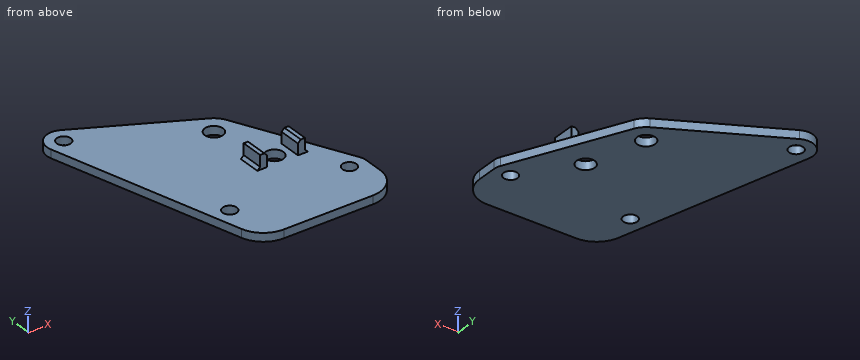
from build123d import *

# Parameters (mm, degrees)
SKETCH1_R           = 2.5
SKETCH1_R_2         = 3.25
BOSS_EXTRUDE1_DEPTH = 3
SKETCH2_W           = 2.5
SKETCH2_H           = 8
BOSS_EXTRUDE2_DEPTH = 5
CHAMFER1_SIZE       = 1
FILLET1_R           = 10


with BuildPart() as part:
    # Sketch1 → Boss-Extrude1 (new body)
    with BuildSketch(Plane.XY):
        with BuildLine():
            Line((-63.791318359, 58.43135993), (-43.395591792, -16.868352188))
            Line((-43.395591792, -16.868352188), (6, -16.868352188))
            Line((6, -16.868352188), (6, 0))
            ThreePointArc((6, 0), (5.850545761, 1.330832182), (5.409628568, 2.595364861))
            Line((5.409628568, 2.595364861), (-13.395576429, 41.791847675))
            ThreePointArc((-13.395576429, 41.791847675), (-14.765199318, 43.760307326), (-16.686113759, 45.195851809))
            Line((-16.686113759, 45.195851809), (-55.222801296, 65.318568168))
            ThreePointArc((-55.222801296, 65.318568168), (-61.758941161, 64.676575814), (-63.791318359, 58.43135993))
        make_face()
        Circle(SKETCH1_R, mode=Mode.SUBTRACT)
        with Locations((-58, 60)):
            Circle(SKETCH1_R, mode=Mode.SUBTRACT)
        with Locations((-42, 0.929027955)):
            Circle(SKETCH1_R, mode=Mode.SUBTRACT)
        with Locations((-20.157612139, 38.547641599)):
            Circle(SKETCH1_R_2, mode=Mode.SUBTRACT)
        with Locations((-13.798527561, 17.748013157)):
            Circle(SKETCH1_R_2, mode=Mode.SUBTRACT)
    extrude(amount=BOSS_EXTRUDE1_DEPTH)

    # Sketch2 → Boss-Extrude2 (add)
    with BuildSketch(Plane.XY.offset(3)):
        with Locations((-7.048527561, 17.748013157)):
            Rectangle(SKETCH2_W, SKETCH2_H)
        with Locations((-20.548527561, 17.748013157)):
            Rectangle(SKETCH2_W, SKETCH2_H)
    extrude(amount=BOSS_EXTRUDE2_DEPTH)

    # Chamfer1
    chamfer1_edges = [part.edges().sort_by_distance(p)[0] for p in [
        (-5.798527561, 17.748013157, 3),
        (-8.298527561, 17.748013157, 8),
        (-21.798527561, 17.748013157, 3),
        (-19.298527561, 17.748013157, 8),
    ]]
    chamfer(chamfer1_edges, length=CHAMFER1_SIZE)

    # Fillet1
    fillet1_edges = [part.edges().sort_by_distance(p)[0] for p in [
        (6, -16.868352188, 1.5),
        (-43.395591792, -16.868352188, 1.5),
    ]]
    fillet(fillet1_edges, radius=FILLET1_R)


solid = part.part
Check sheet for the modelled part. Datum: model origin and axes. Units: mm. Give positions to 0.01 mm unless a question says otherwise; leave off trailing zeros. Loops run counter-clockwise (first coordinate to the right, second up) from the corner with the lowest first, then second, coordinate; pieces in that order, holes last. Notation, with made-up numbers: M 12,21 L 66,21 A17 cw 66,53 Z; hole C 20,-30 d2. An arc over 180 degrees is marked long. Answer as a JSON object with one key per item and string values. Group by question number.
Q1. Go/stop test with flat-tipped pins: P1, Ø8.5, axis at x = -13.8, y = 17.75, coming from the +Z side; P2, Ø3, axis at x = -22, z = 5, coming from the +Y side; P3, Ø3, axis at y = -4.5, z = 1, coming from the -X side. Record where each tip stops, or that it passes through.
Q2. Cross-section at D-D on x = -34. Record the cut outline in (y, z).
Q3. Cross-section at A-A on x = -42. Record the cut outline in (y, z).
Q4. Material ranges on line 1 along Z through (x, y) = (-3, -9); line 2 along Y through (x, z) = (-15, 1.5); line 3 along X through (y, z) = (39, 2.5), recorded low to high. Write a range as [from, to].
Q5. Cross-section at C-C on y = 54.5. Record the cut outline in (x, z), then the cut area to 3 significant figures.
Q6. Cross-section at B-B on y = 37. Record the cut outline in (x, z).
Evaluation:
{
 "1": {"P1": "stops at z = 3", "P2": "stops at y = 21.75", "P3": "stops at x = -47.15"},
 "2": {"outline": "M -16.87,0 L 54.24,0 L 54.24,3 L -16.87,3 Z"},
 "3": {"outline": "M -14.67,0 L -1.57,0 L -1.57,3 L -14.67,3 Z; M 3.43,0 L 58.41,0 L 58.41,3 L 3.43,3 Z"},
 "4": {"line 1": "z = [0, 3]", "line 2": "y = [-16.87, 14.73], [20.77, 43.99]", "line 3": "x = [-58.53, -23.38], [-16.94, -12.06]"},
 "5": {"outline": "M -62.73,0 L -34.5,0 L -34.5,3 L -62.73,3 Z", "area": "84.7 mm2"},
 "6": {"outline": "M -57.99,0 L -23.02,0 L -23.02,3 L -57.99,3 Z; M -17.3,0 L -11.1,0 L -11.1,3 L -17.3,3 Z"}
}
